CAD build for the part. Positions are in the model's coordinates, mm. Coordinates: 2 decimals unless noted, no trailing zeros. Write each loop counter-clockwise with the first axis right and the second up, starting at its lowest first coordinate (ties: lowest second). Pieces come first, ordered by that corner, then holes.
```python
from build123d import *

# Parameters (mm, degrees)
F0_R     = 9
F0_R_2   = 1.5
F1_DEPTH = 25


with BuildPart() as f1:
    # F0 (on Top) → F1 (new body)
    with BuildSketch(Plane.XY):
        Circle(F0_R)
        with Locations((-7, 0)):
            Circle(F0_R_2, mode=Mode.SUBTRACT)
        with BuildLine():
            ThreePointArc((-1.25, 5.25), (0, 6.5), (1.25, 5.25))
            Line((1.25, 5.25), (1.25, -5.25))
            ThreePointArc((1.25, -5.25), (0, -6.5), (-1.25, -5.25))
            Line((-1.25, -5.25), (-1.25, 5.25))
        make_face(mode=Mode.SUBTRACT)
        with Locations((7, 0)):
            Circle(F0_R_2, mode=Mode.SUBTRACT)
    extrude(amount=F1_DEPTH)


solid = f1.part
```
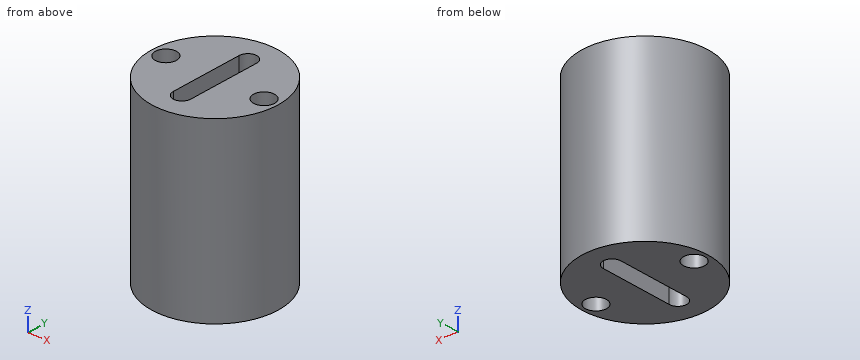
Item 1: Saw through at C-C, the plane z = 6. Write the cut outline in (x, y).
Item 2: Wall check: line 1 along X through (y, z) = (-0.25, 6.5); line 2 along X through (y, z) = (3.5, 12.25); line 3 along X through (y, z) = (-5.75, 13.25). Give the ranges that are in metal, low to high.
Item 3: Saw through at B-B, the plane x = 0. Write the cut outline in (y, z).
Item 4: Saw through at D-D, the plane y = -3.5. Write the cut outline in (x, z), and give its area (3 significant figures).
Item 5: Saw through at A-A, the plane y = 0. Write the cut outline in (x, z), and give its area (4 significant figures).
Item 6: Flat gauge pins, fed straight in: pin 1 Ø5 at (y, z) = (-4.5, 12.5) entering from -X; pin 2 Ø6 at (x, z) = (-5, 9) entering from +Y; pin 3 Ø1 at (x, z) = (3, 19.5) entering from +Y. Where does each tip first touch, or does it go through?
Working result:
1. outline: circle Ø18 at (0, 0); hole circle Ø3 at (-7, 0); hole (-1.25, -5.25) arc R1.25 ccw to (1.25, -5.25) - (1.25, 5.25) arc R1.25 ccw to (-1.25, 5.25) - close; hole circle Ø3 at (7, 0)
2. line 1: x = -9 to -8.48, -5.52 to -1.25, 1.25 to 5.52, 8.48 to 9
2. line 2: x = -8.29 to -1.25, 1.25 to 8.29
2. line 3: x = -6.92 to -1.15, 1.15 to 6.92
3. outline: (-9, 0) - (-6.5, 0) - (-6.5, 25) - (-9, 25) - close; (6.5, 0) - (9, 0) - (9, 25) - (6.5, 25) - close
4. outline: (-8.29, 0) - (-1.25, 0) - (-1.25, 25) - (-8.29, 25) - close; (1.25, 0) - (8.29, 0) - (8.29, 25) - (1.25, 25) - close
4. area: 352 mm2
5. outline: (-9, 0) - (-8.5, 0) - (-8.5, 25) - (-9, 25) - close; (-5.5, 0) - (-1.25, 0) - (-1.25, 25) - (-5.5, 25) - close; (1.25, 0) - (5.5, 0) - (5.5, 25) - (1.25, 25) - close; (8.5, 0) - (9, 0) - (9, 25) - (8.5, 25) - close
5. area: 237.5 mm2
6. pin 1: stops at x = -8.77
6. pin 2: stops at y = 8.77
6. pin 3: stops at y = 8.65
